Geometry: final body of the model. Coordinates: model frame, mm. Face numbers are marked on the shaded views. A direction names the side the tool comes from. Coordinates: 2 decimals unless noted, no trailing zeros. Loops run counter-clockwise (first coordinate to the right, second up) from the corner with the lowest first, then second, coordinate; pieces in that order, holes last. Notation, with made-up numbers: (-27.75, 58) - (21.25, 58) arc R32 cw to (21.25, 89) - close; hole circle Ø3 at (-6.75, 20.5). An arc over 180 degrees is marked (long way). Put each result on its own line as item: value. Start each with the question number.
1) Section B-B on z = 8. Output: boundary loops of the cut face in (x, y), and give its area (3 significant figures).
2) Section A-A on y = 3.25. Output: boundary loops of the cut face in (x, z), and give its area (3 significant figures).
3) Draft query along X for the marked faces 3, 4, 5 and 6. Return one class per face: +X half, -X half, draft (parallel to the pull), parting line (faces both ways), or undercut.
4) Reachability of the marked faces 1 and 2 from +Z, -Z, +X, -X, +Y, -Y: full face, straight path, thin tool, end or side. Return the list, or none.
5) Section C-C on x = -8. Output: boundary loops of the cut face in (y, z), and give its area (3 significant figures).
6) Material intervals for line 1 along Y through (x, z) = (-3.5, 9); line 2 along Y through (x, z) = (11, 7.75); line 3 along X through (y, z) = (6.25, 7.75), sorted ascending. Write a range as from..to.
7) Contact query for flat-ended pins moving along their axis: pin 1 Ø1.8 at (x, y) = (-14.66, -5.66) entering from +Z; pin 2 Ø1.5 at (y, z) = (1.5, 5) entering from -X. Output: stop coordinate, or through.
8) Section D-D on x = -15. Output: boundary loops of the cut face in (y, z), and give its area (3 significant figures).
```python
from build123d import *

# Parameters (mm, degrees)
F0_R     = 1.5
F0_R_2   = 5.1
F1_DEPTH = 10


with BuildPart() as f1:
    # F0 (on Top) → F1 (new body)
    with BuildSketch(Plane.XY):
        with BuildLine():
            ThreePointArc((20, 5.1), (18.27193, 9.27193), (14.1, 11))
            Line((14.1, 11), (-9, 11))
            ThreePointArc((-9, 11), (-16.778175, 7.778175), (-20, 0))
            ThreePointArc((-20, 0), (-16.778175, -7.778175), (-9, -11))
            Line((-9, -11), (14.1, -11))
            ThreePointArc((14.1, -11), (18.27193, -9.27193), (20, -5.1))
            Line((20, -5.1), (10.1, -5.1))
            ThreePointArc((10.1, -5.1), (6.493755, -3.606245), (5, 0))
            ThreePointArc((5, 0), (6.493755, 3.606245), (10.1, 5.1))
            Line((10.1, 5.1), (20, 5.1))
        make_face()
        with Locations((-14.656854, -5.656854)):
            Circle(F0_R, mode=Mode.SUBTRACT)
        with Locations((-3.343146, -5.656854)):
            Circle(F0_R, mode=Mode.SUBTRACT)
        with Locations((-9, 0)):
            Circle(F0_R_2, mode=Mode.SUBTRACT)
        with Locations((-14.656854, 5.656854)):
            Circle(F0_R, mode=Mode.SUBTRACT)
        with Locations((-3.343146, 5.656854)):
            Circle(F0_R, mode=Mode.SUBTRACT)
    extrude(amount=F1_DEPTH)


solid = f1.part
```
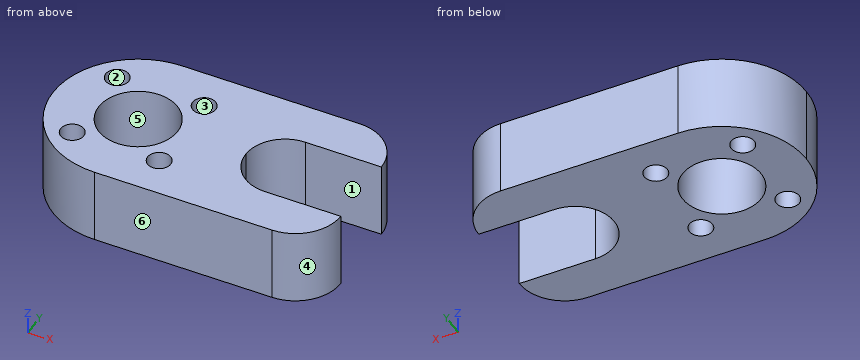
Answer block:
1. outline: (-20, 0) arc R11 ccw to (-9, -11) - (14.1, -11) arc R5.9 ccw to (20, -5.1) - (10.1, -5.1) arc R5.1 cw to (5, 0) arc R5.1 cw to (10.1, 5.1) - (20, 5.1) arc R5.9 ccw to (14.1, 11) - (-9, 11) arc R11 ccw to start; hole circle Ø3 at (-14.66, -5.66); hole circle Ø3 at (-14.66, 5.66); hole circle Ø10.2 at (-9, 0); hole circle Ø3 at (-3.34, -5.66); hole circle Ø3 at (-3.34, 5.66)
1. area: 561 mm²
2. outline: (-19.51, 0) - (-12.93, 0) - (-12.93, 10) - (-19.51, 10) - close; (-5.07, 0) - (6.17, 0) - (6.17, 10) - (-5.07, 10) - close
2. area: 178 mm²
3. face 3: undercut
3. face 4: +X half
3. face 5: undercut
3. face 6: draft
4. face 1: +Z, -Z, +X
4. face 2: +Z, -Z
5. outline: (-11, 0) - (-5, 0) - (-5, 10) - (-11, 10) - close; (5, 0) - (11, 0) - (11, 10) - (5, 10) - close
5. area: 120 mm²
6. line 1: y = -11..-7.15, -4.17..4.17, 7.15..11
6. line 2: y = -11..-5.1, 5.1..11
6. line 3: x = -18.05..-16.03, -13.28..-4.72, -1.97..19.89
7. pin 1: passes through
7. pin 2: stops at x = -19.97
8. outline: (-9.22, 0) - (-7.12, 0) - (-7.12, 10) - (-9.22, 10) - close; (-4.2, 0) - (4.2, 0) - (4.2, 10) - (-4.2, 10) - close; (7.12, 0) - (9.22, 0) - (9.22, 10) - (7.12, 10) - close
8. area: 126 mm²
